Can you work these out from the model? Positions are in its coordinate system, mm. Face numbers are marked on the shaded views. A direction names the side the tool comes from. Give positions to 0.01 mm unless a question says otherwise; leave off trailing zeros. Order: outer loops, then holes, each group sorted by start corner. A loop starts at its lowest first (then second) coordinate and runs counter-clockwise, first axis right, second up. Notation, with made-up numbers: M 4,-36 L 61,-36 A20 cw 61,-5 Z; hole C 19,-1.75 d2. An arc over 180 degrees is marked long. Answer as a JSON object with one key per item and string values.
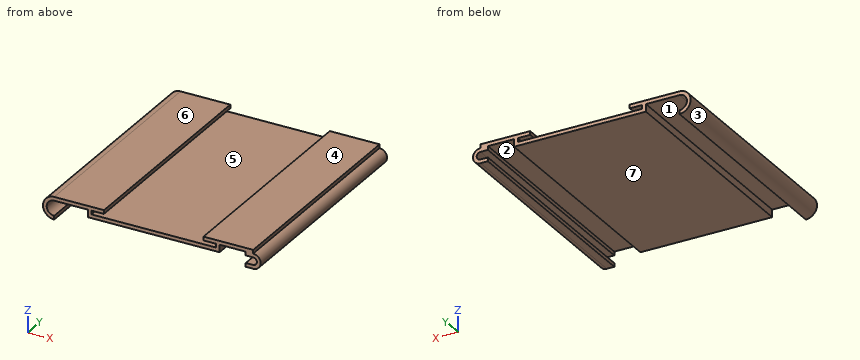
```python
from build123d import *

# Parameters (mm, degrees)
F1_DEPTH  = 90
F2_W      = 50
F2_H      = 3
F3_DEPTH  = 90.001
F4_T      = -1.5
F6_DEPTH  = 90.001
F7_W      = 5
F7_H      = 1.5
F8_DEPTH  = 90
F10_DEPTH = 90.001


with BuildPart() as f1:
    # F0 (on Front) → F1 (new body)
    with BuildSketch(Plane.XZ):
        with BuildLine():
            ThreePointArc((40.0000004103, -4.5), (44.4999995897, 4.103e-07), (39.9999995897, 4.5))
            Line((39.9999995897, 4.5), (-40.0000004103, 4.5))
            ThreePointArc((-40.0000004103, 4.5), (-44.5000004103, -4.103e-07), (-39.9999995897, -4.5))
            Line((-39.9999995897, -4.5), (40.0000004103, -4.5))
        make_face()
    extrude(amount=F1_DEPTH)

    # F2 (on Front) → F3 (cut, through all)
    with BuildSketch(Plane.XZ):
        with Locations((-4.103e-07, 3)):
            Rectangle(F2_W, F2_H)
    extrude(amount=F3_DEPTH, mode=Mode.SUBTRACT)

    # F4
    f4_openings = [f1.faces().sort_by_distance(p)[0] for p in [
        (0, -90, -0.710208),
        (0, 0, -0.710208),
    ]]
    offset(amount=F4_T, openings=f4_openings, kind=Kind.INTERSECTION)

    # F5 (on Front) → F6 (cut, through all)
    with BuildSketch(Plane.XZ):
        with BuildLine():
            ThreePointArc((39.9999995897, 3), (42.9999995897, 4.103e-07), (40.0000004103, -3))
            Line((40.0000004103, -3), (-39.9999998632, -3))
            Line((-39.9999998632, -3), (-39.9999995897, -4.5))
            Line((-39.9999995897, -4.5), (40.0000004103, -4.5))
            ThreePointArc((40.0000004103, -4.5), (44.4999995897, 4.103e-07), (39.9999995897, 4.5))
            Line((39.9999995897, 4.5), (39.9999995897, 3))
        make_face()
    extrude(amount=F6_DEPTH, mode=Mode.SUBTRACT)

    # F7 (on Front) → F8 (join, through all)
    with BuildSketch(Plane.XZ):
        with BuildLine():
            Line((36.9999995897, -3), (39.9999995897, -3))
            ThreePointArc((39.9999995897, -3), (42.9999995897, 0), (39.9999995897, 3))
            Line((39.9999995897, 3), (36.9999995897, 3))
            Line((36.9999995897, 3), (36.9999995897, 0))
            Line((36.9999995897, 0), (36.9999995897, -3))
        make_face()
        with Locations((-22.5000004103, 3.75)):
            Rectangle(F7_W, F7_H)
        with Locations((22.5000004103, 3.75)):
            Rectangle(F7_W, F7_H)
    extrude(amount=F8_DEPTH)

    # F9 (on Front) → F10 (cut, through all)
    with BuildSketch(Plane.XZ):
        with BuildLine():
            Line((36.9999995897, -1.5), (39.9999995897, -1.5))
            ThreePointArc((39.9999995897, -1.5), (41.4999995897, 0), (39.9999995897, 1.5))
            Line((39.9999995897, 1.5), (36.9999995897, 1.5))
            Line((36.9999995897, 1.5), (36.9999995897, -1.5))
        make_face()
    extrude(amount=F10_DEPTH, mode=Mode.SUBTRACT)


solid = f1.part
```
1) For the marked faces 5, 6 and 7, which set-ups out of +Z, -Z, +X, -X, +Y, -Y let a thin tool reach every point of the face, with its end or its side?
Results found:
{"face 5": "+Y, -Y", "face 6": "+Z, +X, -X, +Y, -Y", "face 7": "-Z, +Y, -Y"}
2) Thinking about a two-plate mould opening in X: for the marked faces 1, 2, 3 and 4, which applies, pulls with the +X half, pulls with the -X half, needs draft (parallel to the pull), parting line crosses it, or undercut?
Results found:
{"face 1": "undercut", "face 2": "undercut", "face 3": "pulls with the -X half", "face 4": "needs draft"}
3) I need wall thicknesses on L1, parallel to Z at x = -21, y = -24; L2, parallel to Z at x = 35, y = -74; L3, parallel to X at y = -10, z = 3.75. Which ranges of each line are inside material? Lowest first, please.
Results found:
{"L1": "z = 0 to 1.5, 3 to 4.5", "L2": "z = 3 to 4.5", "L3": "x = -42.49 to -20, 20 to 40"}
4) I'm going to push flat-ended pins straight in: pin 1 Ø1.2 at (y, z) = (-56.5, -4) entering from +X; pin 2 Ø1.6 at (y, z) = (-45, 2.5) entering from -X; pin 3 Ø1.2 at (y, z) = (-48.5, 2) entering from -X. Where does each tip first touch, or does it pass through?
Results found:
{"pin 1": "stops at x = -40", "pin 2": "stops at x = -44.17", "pin 3": "stops at x = -44.28"}
5) I want a section at B-B on x = -31. Write out the boundary of the cut face in (y, z).
Results found:
{"outline": "M -90,3 L 0,3 L 0,4.5 L -90,4.5 Z"}
6) I want a section at A-A on y = -8. Write out the boundary of the cut face in (x, z), and give its area (3 significant figures).
Results found:
{"outline": "M -40,-4.5 L -40,-3 A3 cw -40,3 L -26.5,3 L -26.5,0 L 26.5,0 L 26.5,3 L 37,3 L 37,1.5 L 40,1.5 A1.5 cw 40,-1.5 L 37,-1.5 L 37,-3 L 40,-3 A3 ccw 40,3 L 40,4.5 L 20,4.5 L 20,3 L 25,3 L 25,1.5 L -25,1.5 L -25,3 L -20,3 L -20,4.5 L -40,4.5 A4.5 ccw Z", "area": "181 mm²"}
